The figure shows three views and two pictorial views of one solid part (mm, origin at its lowest corner). Answer the questions. Round coordinates to 2 decimals unless told otherwise and drop trailing zeros. Order: outer loops, then holes, each group sorted by start corner. A loop starts at its lowest first (then second) coordinate and runs counter-clockwise, first axis right, second up. Notation, with made-up numbers: (57, 52) -> (87, 52) arc R31 cw to (87, 87) -> close; hole circle Ø10 at (33.25, 36). An arc over 180 degrees is marked (long way). One line per item, written item: value. Start each with the question number.
1. Section C-C (y = 24.5) is taken. Give the vertices of the cut face in (x, z), then the cut area to 3 significant figures.
2. Section B-B (z = 0.4) is taken. Give the vertices of the cut face in (x, y), then the cut area to 3 significant figures.
3. A flat-ended cylindrical pin translates along its axis: pin 1 Ø10 at (x, y) = (31.5, 79.5) entering from +Z. Find the tip coordinate at first contact, or state that the pin passes through.
4. Section A-A (x = 66) is taken. Give the vertices of the cut face in (y, z), then the cut area to 3 significant figures.
5. Section D-D (y = 74.5) is taken. Give the vertices of the cut face in (x, z), then the cut area to 3 significant figures.
6. Consider line 1 (Y direction, x = 66, z = 1.6); line 2 (X direction, y = 66, z = 1.35); line 3 (X direction, y = 27.1, z = 0.65) (1 decimal). Determine where each line is inside the solid, lowest interval first.
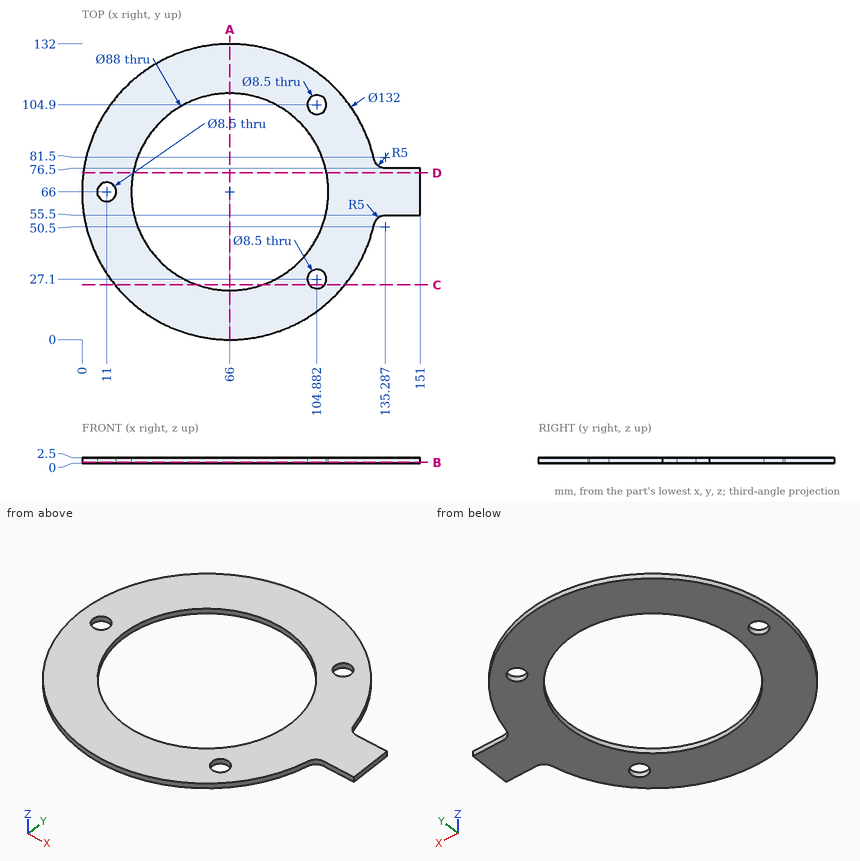
Answer:
1. outline: (14.68, 0) -> (51.38, 0) -> (51.38, 2.5) -> (14.68, 2.5) -> close; (80.62, 0) -> (101.52, 0) -> (101.52, 2.5) -> (80.62, 2.5) -> close; (108.24, 0) -> (117.32, 0) -> (117.32, 2.5) -> (108.24, 2.5) -> close
1. area: 167 mm^2
2. outline: (130.41, 51.59) arc R5 cw to (135.29, 55.5) -> (151, 55.5) -> (151, 76.5) -> (135.29, 76.5) arc R5 cw to (130.41, 80.41) arc R66 ccw (long way) to start; hole circle Ø8.5 at (11, 66); hole circle Ø88 at (66, 66); hole circle Ø8.5 at (104.88, 27.1); hole circle Ø8.5 at (104.88, 104.9)
2. area: 7,840 mm^2
3. pin 1: through
4. outline: (0, 0) -> (22, 0) -> (22, 2.5) -> (0, 2.5) -> close; (110, 0) -> (132, 0) -> (132, 2.5) -> (110, 2.5) -> close
4. area: 110 mm^2
5. outline: (0.55, 0) -> (22.83, 0) -> (22.83, 2.5) -> (0.55, 2.5) -> close; (109.17, 0) -> (151, 0) -> (151, 2.5) -> (109.17, 2.5) -> close
5. area: 160 mm^2
6. line 1: 0 to 22, 110 to 132
6. line 2: 0 to 6.75, 15.25 to 22, 110 to 151
6. line 3: 12.7 to 45.4, 86.6 to 100.6, 109.1 to 119.3
